from build123d import *

# Parameters (mm, degrees)
F1_DEPTH = 3.81
F3_DEPTH = 3.81
F5_DEPTH = 3.81


with BuildPart() as f1:
    # F0 (on Top) → F1 (new body)
    with BuildSketch(Plane.XY):
        with BuildLine():
            Line((16.97628, -59.058286), (19.705089, -52.957691))
            Line((19.705089, -52.957691), (31.07564, -43.799512))
            ThreePointArc((31.07564, -43.799512), (33.366016, -43.816918), (35.622127, -44.211995))
            Line((35.622127, -44.211995), (36.541499, -43.411601))
            Line((36.541499, -43.411601), (39.299611, -43.411601))
            Line((39.299611, -43.411601), (39.659975, -43.95369))
            Line((39.659975, -43.95369), (38.401872, -44.655453))
            Line((38.401872, -44.655453), (36.541499, -50.125077))
            Line((36.541499, -50.125077), (41.410863, -48.1015))
            Line((41.410863, -48.1015), (41.462618, -48.226037))
            Line((41.462618, -48.226037), (43.122184, -48.226037))
            Line((43.122184, -48.226037), (41.909318, -52.580997))
            Line((41.909318, -52.580997), (46.375882, -50.965246))
            ThreePointArc((46.375882, -50.965246), (50.990398, -50.455311), (55.107314, -48.309434))
            ThreePointArc((55.107314, -48.309434), (55.96993, -45.777959), (55.834934, -43.106958))
            Line((55.834934, -43.106958), (57.362933, -43.106958))
            Line((57.362933, -43.106958), (56.926362, -48.454959))
            Line((56.926362, -48.454959), (60.218841, -45.999244))
            Line((60.218841, -45.999244), (60.455315, -46.708673))
            Line((60.455315, -46.708673), (64.166173, -42.397529))
            ThreePointArc((64.166173, -42.397529), (65.729722, -42.177688), (66.959918, -41.187923))
            ThreePointArc((66.959918, -41.187923), (67.726373, -38.917492), (69.034263, -36.909573))
            ThreePointArc((69.034263, -36.909573), (71.467629, -31.352581), (71.514241, -25.286343))
            ThreePointArc((71.514241, -25.286343), (68.607951, -22.424523), (64.549089, -22.021808))
            ThreePointArc((64.549089, -22.021808), (62.040176, -19.042247), (58.826987, -16.840467))
            ThreePointArc((58.826987, -16.840467), (53.707685, -17.118566), (48.670236, -18.071821))
            ThreePointArc((48.670236, -18.071821), (41.311862, -21.003722), (34.429371, -24.924567))
            Line((34.429371, -24.924567), (33.67985, -24.924567))
            ThreePointArc((33.67985, -24.924567), (27.48786, -28.135727), (21.901691, -32.312687))
            Line((21.901691, -32.312687), (10.765978, -33.169281))
            Line((10.765978, -33.169281), (5.733491, -43.127179))
            Line((5.733491, -43.127179), (17.939948, -41.628141))
            Line((17.939948, -41.628141), (10.873053, -49.658701))
            Line((10.873053, -49.658701), (8.731569, -52.978002))
            Line((8.731569, -52.978002), (7.653544, -56.265509))
            Line((7.653544, -56.265509), (10.765978, -60.044896))
            Line((10.765978, -60.044896), (14.075343, -53.394235))
            Line((14.075343, -53.394235), (14.600779, -54.032265))
            Line((14.600779, -54.032265), (13.549907, -54.897688))
            Line((13.549907, -54.897688), (16.97628, -59.058286))
        make_face()
    extrude(amount=F1_DEPTH)

    # F2 (on face) → F3 (join)
    with BuildSketch(Plane(origin=(0, 0, 0), x_dir=(1, 0, 0), z_dir=(0, 0, -1))):
        with BuildLine():
            Line((62.362719, 21.262165), (64.074621, 23.344252))
            ThreePointArc((64.074621, 23.344252), (67.036734, 23.376149), (69.694884, 24.683576))
            ThreePointArc((69.694884, 24.683576), (70.644255, 27.084462), (70.225157, 29.631993))
            ThreePointArc((70.225157, 29.631993), (69.955998, 33.029778), (68.25655, 35.984311))
            ThreePointArc((68.25655, 35.984311), (67.0841, 38.480973), (65.636583, 40.828876))
            ThreePointArc((65.636583, 40.828876), (64.574593, 41.408491), (63.365407, 41.449059))
            Line((63.365407, 41.449059), (61.005343, 44.63305))
            Line((61.005343, 44.63305), (60.600822, 44.333207))
            Line((60.600822, 44.333207), (58.44954, 46.232879))
            Line((58.44954, 46.232879), (58.757726, 43.257009))
            ThreePointArc((58.757726, 43.257009), (58.639112, 42.628479), (58.195706, 42.167488))
            ThreePointArc((58.195706, 42.167488), (57.966711, 42.031397), (57.721477, 41.927379))
            Line((57.721477, 41.927379), (52.187819, 42.170435))
            ThreePointArc((52.187819, 42.170435), (51.292653, 44.391683), (49.575482, 46.060991))
            ThreePointArc((49.575482, 46.060991), (45.619915, 46.921487), (41.575972, 47.104497))
            Line((41.575972, 47.104497), (38.279213, 48.226037))
            Line((38.279213, 48.226037), (39.414629, 45.300853))
            Line((39.414629, 45.300853), (41.011725, 44.848081))
            Line((41.011725, 44.848081), (41.011725, 43.914717))
            Line((41.011725, 43.914717), (44.32217, 42.485248))
            Line((44.32217, 42.485248), (36.116112, 42.485248))
            Line((36.116112, 42.485248), (35.539597, 43.173272))
            ThreePointArc((35.539597, 43.173272), (26.07418, 43.15441), (17.62064, 47.412593))
            Line((17.62064, 47.412593), (17.572723, 47.698561))
            ThreePointArc((17.572723, 47.698561), (16.460668, 49.519729), (15.021231, 51.094957))
            Line((15.021231, 51.094957), (11.698972, 53.478461))
            Line((11.698972, 53.478461), (9.989955, 57.935085))
            Line((9.989955, 57.935085), (7.880738, 55.572665))
            Line((7.880738, 55.572665), (8.731569, 53.835317))
            Line((8.731569, 53.835317), (8.731569, 52.978002))
            Line((8.731569, 52.978002), (10.910701, 51.094957))
            Line((10.910701, 51.094957), (11.512643, 49.018534))
            ThreePointArc((11.512643, 49.018534), (15.92645, 45.583856), (19.22353, 41.066337))
            Line((19.22353, 41.066337), (19.28794, 40.791228))
            Line((19.28794, 40.791228), (63.54069, 34.192108))
            ThreePointArc((63.54069, 34.192108), (63.531632, 36.09198), (65.42775, 36.21171))
            ThreePointArc((65.42775, 36.21171), (64.621892, 35.279534), (65.201432, 34.192108))
            ThreePointArc((65.201432, 34.192108), (65.613039, 30.902592), (67.980655, 28.582089))
            Line((67.980655, 28.582089), (23.599958, 32.474866))
            Line((23.599958, 32.474866), (34.688797, 26.033277))
            Line((34.688797, 26.033277), (34.380915, 25.503276))
            Line((34.380915, 25.503276), (35.281472, 24.36841))
            ThreePointArc((35.281472, 24.36841), (42.420934, 21.024647), (49.938917, 18.651335))
            Line((49.938917, 18.651335), (50.498281, 18.300841))
            Line((50.498281, 18.300841), (50.135953, 17.722592))
            Line((50.135953, 17.722592), (54.223109, 17.459012))
            Line((54.223109, 17.459012), (54.223109, 17.059586))
            Line((54.223109, 17.059586), (58.015913, 18.300841))
            Line((58.015913, 18.300841), (58.496706, 17.714143))
            Line((58.496706, 17.714143), (60.837945, 19.632767))
            Line((60.837945, 19.632767), (62.362719, 21.262165))
        make_face()
        with BuildLine():
            Line((52.715112, 43.126516), (54.523326, 43.126516))
            ThreePointArc((54.523326, 43.126516), (55.015238, 45.857392), (53.44123, 48.142597))
            Line((53.44123, 48.142597), (53.128958, 48.463933))
            ThreePointArc((53.128958, 48.463933), (49.676827, 49.504967), (46.111207, 50.04099))
            Line((46.111207, 50.04099), (43.576807, 50.933365))
            Line((43.576807, 50.933365), (44.317115, 48.226037))
            ThreePointArc((44.317115, 48.226037), (49.335622, 47.025861), (52.715112, 43.126516))
        make_face()
        with BuildLine():
            Line((18.673604, 52.224013), (16.605122, 57.203803))
            Line((16.605122, 57.203803), (14.549939, 54.708222))
            Line((14.549939, 54.708222), (15.730347, 53.190444))
            Line((15.730347, 53.190444), (15.730347, 52.394051))
            ThreePointArc((15.730347, 52.394051), (17.295057, 51.092122), (18.096911, 49.221195))
            ThreePointArc((18.096911, 49.221195), (23.003501, 45.414789), (29.022919, 43.888368))
            Line((29.022919, 43.888368), (18.673604, 52.224013))
        make_face()
    extrude(amount=F3_DEPTH)

    # F4 (on face) → F5 (join)
    with BuildSketch(Plane(origin=(0, 0, 0), x_dir=(1, 0, 0), z_dir=(0, 0, -1))):
        with BuildLine():
            ThreePointArc((63.215862, 29.757198), (62.30207, 31.580695), (62.900014, 33.530727))
            Line((62.900014, 33.530727), (7.135111, 41.687112))
            Line((7.135111, 41.687112), (11.278112, 34.312829))
            Line((11.278112, 34.312829), (63.215862, 29.757198))
        make_face()
    extrude(amount=F5_DEPTH)


solid = f1.part
For this review, take the finished solid that the model builds, in its own axes (mm). A direction names the side the tool comes from. Give positions to 0.01 mm unless a question says otherwise; leave off trailing zeros. Loops run counter-clockwise (first coordinate to the right, second up) from the corner with the lowest first, then second, coordinate; pieces in that order, holes last. Notation, with made-up numbers: M 82,79.5 L 102,79.5 A25 cw 102,106.5 Z; hole C 71.5,-10.75 d9. An arc over 180 degrees is marked long. Put each result on its own line as item: value. Start each with the question number.
(1) Wall thickness on L1, parallel to X at y = -45, z = 1.5; L2, parallel to X at y = -44.5, z = 0.75; L3, parallel to Y at x = 28, z = -2: over which ranges is each line inside the solid? List them lowest first.
(2) Add section B-B, the plane z = -1. Give the number of separate pieces and of enclosed holes in the cut face, then the cut area to 3 significant figures.
(3) Add section A-A, the plane y = -38. Write out the cut boundary in (x, z), then the cut area to 3 significant figures.
(4) Machinability: for faces 5 (the cylindrical face through (55.023, -45.818, -1.878)), 6 (the flat face through (56.09, -17.67, -1.88)), 7 (the flat face through (57, -43.107, 2)), 8 (the flat face through (9.817, -51.295, 1.878)), which of the approach directions +Z, -Z, +X, -X, +Y, -Y give a long, thin tool a straight path to every point of the face, cutting with its end or side? Answer none if there is none.
(5) The part is to be moulded in two halves that separate along X. For faces 1 (the flat face through (41.1, -37.54, -1.88)), 2 (the cylindrical face through (67.1, -38.45, -1.88)), 3 (the flat face through (34, -32, 0)), 4 (the cylindrical face through (41.412, -20.956, 1.878)), say which applies: +X half, -X half, draft (parallel to the pull), parting line (faces both ways), or undercut.
(6) For pin 1 (2 mm diameter, centred on x = 39, z = 0, fed in from -Y); pin 2 (0.8 mm diameter, centred on x = 34, z = 2.5, fed in from +Y); pin 3 (1.8 mm diameter, centred on x = 42.5, z = 2.5, fed in from -Y); pin 4 (8 mm diameter, centred on x = 56, y = -45, fed in from -Z), all flat-tipped, find the tip position at first contact; note any pin that passes through.
Result:
1. L1: x = 14.97 to 29.59, 38.28 to 56.04, 57.21 to 61.93
1. L2: x = 15.41 to 30.21, 38.68 to 56.03, 57.25 to 62.36
1. L3: y = -44.71 to -43.97, -42.8 to -39.49, -38.64 to -32.85, -32.09 to -29.92
2. separate pieces: 4
2. enclosed holes: 0
2. area: 1,110 mm^2
3. outline: M 8.32,0 L 9.21,0 L 9.21,-3.81 L 32.34,-3.81 L 32.34,0 L 38.01,0 L 38.01,-3.81 L 67.34,-3.81 L 67.34,0 L 68.24,0 L 68.24,3.81 L 8.32,3.81 Z
3. area: 428 mm^2
4. face 5: -Z
4. face 6: -Z, +Y
4. face 7: +Z, -Z
4. face 8: +Z, -Z, -X
5. face 1: undercut
5. face 2: +X half
5. face 3: undercut
5. face 4: -X half
6. pin 1: stops at y = -49.52
6. pin 2: stops at y = -24.92
6. pin 3: stops at y = -52.58
6. pin 4: stops at z = -3.81
